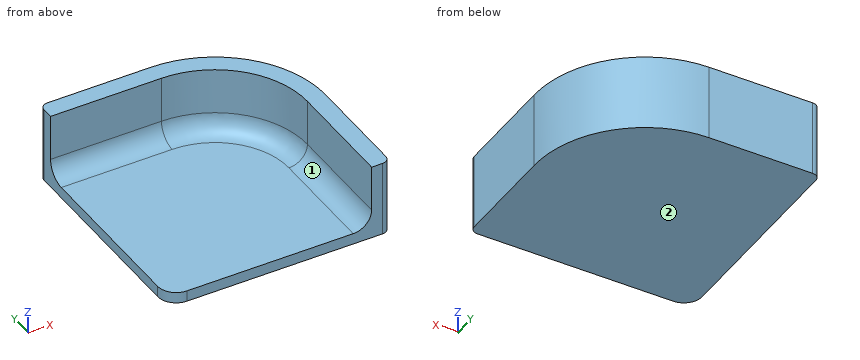
```python
from build123d import *

# Parameters (mm, degrees)
F1_DEPTH = 3
F3_DEPTH = 17.5
F4_R     = 5
F5_R     = 2
F6_R     = 2
F7_R     = 5


with BuildPart() as f1:
    # F0 (on Top) → F1 (new body)
    with BuildSketch(Plane.XY):
        with BuildLine():
            Line((30, 0), (0, 0))
            Line((0, 0), (0, -60))
            Line((0, -60), (60, -60))
            Line((60, -60), (60, -30))
            ThreePointArc((60, -30), (51.2132034356, -8.7867965644), (30, 0))
        make_face()
    extrude(amount=F1_DEPTH)

    # F2 (on face) → F3 (join)
    with BuildSketch(Plane.XY.offset(3)):
        with BuildLine():
            Line((30, 0), (0, 0))
            Line((0, 0), (0, -5))
            Line((0, -5), (30, -5))
            ThreePointArc((30, -5), (47.6776695297, -12.3223304703), (55, -30))
            Line((55, -30), (55, -60))
            Line((55, -60), (60, -60))
            Line((60, -60), (60, -30))
            ThreePointArc((60, -30), (51.2132034356, -8.7867965644), (30, 0))
        make_face()
    extrude(amount=F3_DEPTH)

    # F4
    f4_edges = [f1.edges().sort_by_distance(p)[0] for p in [
        (0, -60, 1.5),
    ]]
    fillet(f4_edges, radius=F4_R)

    # F5
    f5_edges = [f1.edges().sort_by_distance(p)[0] for p in [
        (0, 0, 10.25),
    ]]
    fillet(f5_edges, radius=F5_R)

    # F6
    f6_edges = [f1.edges().sort_by_distance(p)[0] for p in [
        (60, -60, 10.25),
    ]]
    fillet(f6_edges, radius=F6_R)

    # F7
    f7_edges = [f1.edges().sort_by_distance(p)[0] for p in [
        (15, -5, 3),
        (47.67767, -12.32233, 3),
        (55, -45, 3),
    ]]
    fillet(f7_edges, radius=F7_R)


solid = f1.part
```
The listing builds one solid part. Answer for the finished solid, in the listing's coordinates (mm). Face numbers are marked on the shaded views. A direction names the side the tool comes from. Coordinates: 2 decimals unless noted, no trailing zeros. Write each loop counter-clockwise with the first axis right and the second up, starting at its lowest first coordinate (ties: lowest second). Pieces come first, ordered by that corner, then holes. Notation, with made-up numbers: M 66.5,26 L 113.5,26 A18 ccw 113.5,34 Z; hole C 81.25,26 d11. An arc over 180 degrees is marked long. Use a Markdown table: item, result. Add a question column.
1. Section D-D (z = 13) is taken. Give the vertices of the cut face in (x, y).
2. Section A-A (y = -42) is taken. Give the vertices of the cut face in (x, z).
3. Section B-B (x = 14) is taken. Give the vertices of the cut face in (y, z), plus the area to 3 significant figures.
4. Which of the six approach directions +Z, -Z, +X, -X, +Y, -Y give full straight-line access (tool end or side, diameter ignored) to the marked faces 1 and 2?
5. Straight lines are drawn through the part: line 1 along Z through (x, y) = (44.5, -35); line 2 along Y through (x, z) = (28.5, 15.75); line 3 along X through (y, z) = (-34, 16). For each, find the intervals that lie inside material, in ascending order. Write a range as [from, to].
6. Given P1, Ø2, axis at y = -14.5, z = 12, coming from the -X side; P2, Ø6, axis at y = -23, z = 11, coming from the -X side; P3, Ø2, axis at x = 23, y = -52.5, coming from the +Z side, each flat-ended and moving along its own axis, determine where each tip first touches the part or whether it passes through.
7. Section C-C (z = 4) is taken. Give the vertices of the cut face in (x, y).
Data:
| question | item | result |
|---|---|---|
| 1 | outline | M 0,-5 L 30,-5 A25 cw 55,-30 L 55,-60 L 58,-60 A2 ccw 60,-58 L 60,-30 A30 ccw 30,0 L 2,0 A2 ccw 0,-2 Z |
| 2 | outline | M 0,0 L 60,0 L 60,20.5 L 55,20.5 L 55,8 A5 cw 50,3 L 0,3 Z |
| 3 | outline | M -60,0 L 0,0 L 0,20.5 L -5,20.5 L -5,8 A5 cw -10,3 L -60,3 Z |
| 3 | area | 273 mm2 |
| 4 | face 1 | +Z, -X, -Y |
| 4 | face 2 | -Z, +X, -X, +Y, -Y |
| 5 | line 1 | z = [0, 3] |
| 5 | line 2 | y = [-5, 0] |
| 5 | line 3 | x = [55, 60] |
| 6 | P1 | stops at x = 48.78 |
| 6 | P2 | stops at x = 52.91 |
| 6 | P3 | stops at z = 3 |
| 7 | outline | M 0,-7 L 30,-7 A23 cw 53,-30 L 53,-60 L 58,-60 A2 ccw 60,-58 L 60,-30 A30 ccw 30,0 L 2,0 A2 ccw 0,-2 Z |
